Verification items for the finished model (mm, model axes). Face numbers are marked on the shaded views. Round coordinates to 2 decimals unless told otherwise and drop trailing zeros. Write each loop counter-clockwise with the first axis right and the second up, starting at its lowest first coordinate (ties: lowest second). Pieces come first, ordered by that corner, then holes.
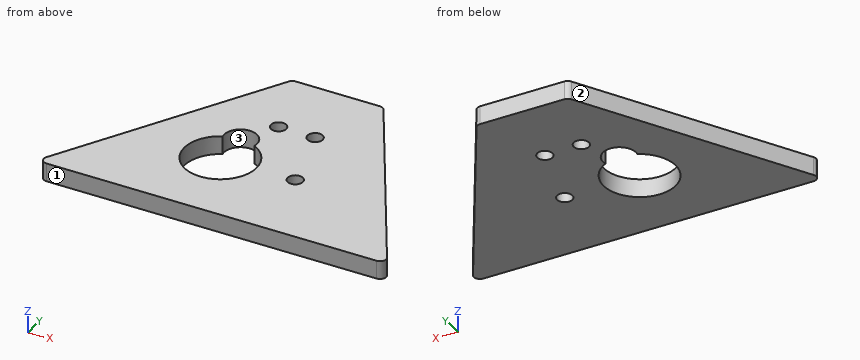
from build123d import *

# Parameters (mm, degrees)
SKETCH001_R      = 2.7
EXTRUDE001_DEPTH = 10
SKETCH_R         = 1.25
SKETCH_R_2       = 5.88
EXTRUDE_DEPTH    = 3
FILLET_R         = 1


with BuildPart() as extrude001:
    # Sketch001 (on Face5 of Fillet) → Extrude001 (new body)
    with BuildSketch(Plane.XY.offset(3)):
        with Locations((-6.109428, 19.36281)):
            Circle(SKETCH001_R)
    extrude(amount=-EXTRUDE001_DEPTH)


with BuildPart() as cut:
    # Sketch → Extrude (new body)
    with BuildSketch(Plane.XY):
        Polygon((0, 0), (28.86196, 0), (7.5, 37), (-7.5, 37), (-28.86196, 0), align=None)
        with Locations((-3, 25)):
            Circle(SKETCH_R, mode=Mode.SUBTRACT)
        with Locations((3, 25)):
            Circle(SKETCH_R, mode=Mode.SUBTRACT)
        with Locations((-6.15, 13.555595)):
            Circle(SKETCH_R_2, mode=Mode.SUBTRACT)
        with Locations((6.15, 13.555595)):
            Circle(SKETCH_R, mode=Mode.SUBTRACT)
    extrude(amount=EXTRUDE_DEPTH)

    # Fillet
    fillet_edges = [cut.edges().sort_by_distance(p)[0] for p in [
        (28.86196, 0, 1.5),
        (7.5, 37, 1.5),
        (-7.5, 37, 1.5),
        (-28.86196, 0, 1.5),
    ]]
    fillet(fillet_edges, radius=FILLET_R)

    # Cut: cut Extrude001
    add(extrude001.part, mode=Mode.SUBTRACT)


solid = cut.part
Q1. Sectioned sample at A-A (x = 3). Enter the section's corners in (y, z).
Recorded:
outline: (0, 0) - (23.75, 0) - (23.75, 3) - (0, 3) - close; (26.25, 0) - (37, 0) - (37, 3) - (26.25, 3) - close
Q2. Sectioned sample at D-D (y = 25). Enter the section's corners in (x, z), plus the area to 3 significant figures.
Recorded:
outline: (-14.43, 0) - (-4.25, 0) - (-4.25, 3) - (-14.43, 3) - close; (-1.75, 0) - (1.75, 0) - (1.75, 3) - (-1.75, 3) - close; (4.25, 0) - (14.43, 0) - (14.43, 3) - (4.25, 3) - close
area: 71.6 mm2
Q3. Sectioned sample at B-B (y = 16.5). Enter the section's corners in (x, z), plus the area to 3 significant figures.
Recorded:
outline: (-19.34, 0) - (-11.24, 0) - (-11.24, 3) - (-19.34, 3) - close; (-1.06, 0) - (19.34, 0) - (19.34, 3) - (-1.06, 3) - close
area: 85.5 mm2
Q4. Release check for a two-part mould opening along X. For the marked faces 1, 2 and 3 record: released by +X, released by -X, zero draft, split by the parting line, or undercut.
Recorded:
face 1: zero draft
face 2: released by -X
face 3: undercut
Q5. Material ranges on line 1 along Y through (x, z) = (-3, 2.1); line 2 along Y through (x, z) = (6.15, 1.3); line 3 along Y through (x, z) = (-6.15, 1.9), recorded low to high.
Recorded:
line 1: y = 0 to 8.59, 18.52 to 23.75, 26.25 to 37
line 2: y = 0 to 12.31, 14.81 to 37
line 3: y = 0 to 7.68, 22.06 to 37
Q6. Sectioned sample at C-C (z = 2.05). Enter the section's corners in (x, y).
Recorded:
outline: (-28, 1.5) arc R1 ccw to (-27.13, 0) - (27.13, 0) arc R1 ccw to (28, 1.5) - (7.79, 36.5) arc R1 ccw to (6.92, 37) - (-6.92, 37) arc R1 ccw to (-7.79, 36.5) - close; hole (-8.76, 18.83) arc R5.88 ccw (long way) to (-3.47, 18.79) arc R2.7 ccw (long way) to start; hole circle Ø2.5 at (-3, 25); hole circle Ø2.5 at (3, 25); hole circle Ø2.5 at (6.15, 13.56)
Q7. Depth check by flat-ended pin: P1, Ø1, axis at x = 15, z = 2, coming from the +Y side. Enter the tip coordinate at first touch or a pass-through.
Recorded:
P1: stops at y = 24.88
